Can you work these out from the drawing? Everything is in mm from the part's minimum corner. Coordinates: 2 decimals unless noted, no trailing zeros. Loops run counter-clockwise (first coordinate to the right, second up) from the corner with the lowest first, then second, coordinate; pieces in that order, holes last.
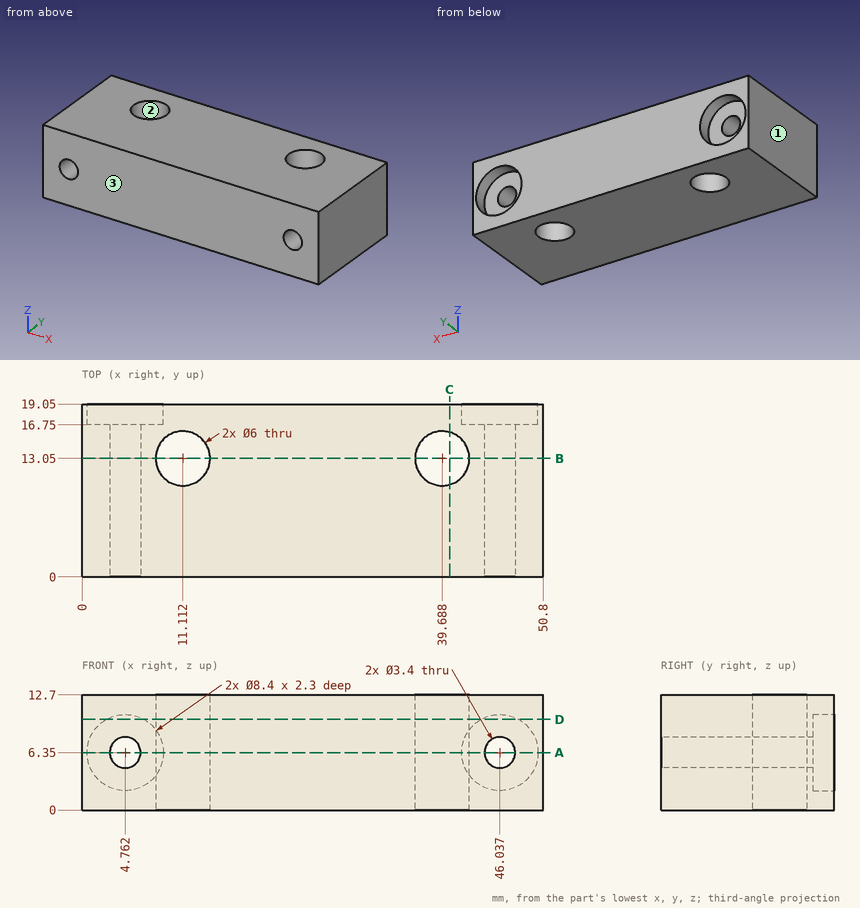
Item 1: I need wall thicknesses on line 1 along X through (y, z) = (2.75, 7.25) (1 decimal); line 2 along X through (y, z) = (14, 5.5) (1 decimal); line 3 along X through (y, z) = (18.25, 2.5) (1 decimal). Which ranges of each line are inside material? Lowest first, please.
Results are:
line 1: x = 0 to 3.3, 6.2 to 44.6, 47.5 to 50.8
line 2: x = 0 to 3.3, 6.2 to 8.3, 14 to 36.8, 42.5 to 44.6, 47.5 to 50.8
line 3: x = 0 to 3.1, 6.4 to 44.4, 47.7 to 50.8
Item 2: Suppose I cut it at A-A, the plane z = 6.35. Please give me the cut outline in (x, y).
Results are:
outline: (0, 0) - (3.06, 0) - (3.06, 16.75) - (0.56, 16.75) - (0.56, 19.05) - (0, 19.05) - close; (6.46, 0) - (44.34, 0) - (44.34, 16.75) - (41.84, 16.75) - (41.84, 19.05) - (8.96, 19.05) - (8.96, 16.75) - (6.46, 16.75) - close; (47.74, 0) - (50.8, 0) - (50.8, 19.05) - (50.24, 19.05) - (50.24, 16.75) - (47.74, 16.75) - close; hole circle Ø6 at (11.11, 13.05); hole circle Ø6 at (39.69, 13.05)
Item 3: Suppose I cut it at D-D, the plane z = 10. Count the separate pieces of the cut face and the enclosed holes in it, plus the area to 3 significant figures.
Results are:
separate pieces: 1
enclosed holes: 2
area: 892 mm2
Item 4: Suppose I cut it at C-C, the plane x = 40.5. Please give me the cut outline in (y, z).
Results are:
outline: (0, 0) - (10.16, 0) - (10.16, 12.7) - (0, 12.7) - close; (15.94, 0) - (19.05, 0) - (19.05, 12.7) - (15.94, 12.7) - close
Item 5: We'd pull the mould along Y, two halves only. Please class the marked faces 1, 2 and 3: +Y half, -Y half, draft (parallel to the pull), parting line (faces both ways), or undercut.
Results are:
face 1: draft
face 2: undercut
face 3: -Y half
Item 6: I'm going to push flat-ended pins straight in: P1, Ø9.5, axis at x = 39.69, y = 13.05, coming from the +Z side; P2, Ø4, axis at x = 45.5, z = 7, coming from the +Y side. Where does each tip first touch, or does it pass through?
Results are:
P1: stops at z = 12.7
P2: stops at y = 16.75
Item 7: Suppose I cut it at B-B, the plane y = 13.05. Please give me the cut outline in (x, z).
Results are:
outline: (0, 0) - (8.11, 0) - (8.11, 12.7) - (0, 12.7) - close; (14.11, 0) - (36.69, 0) - (36.69, 12.7) - (14.11, 12.7) - close; (42.69, 0) - (50.8, 0) - (50.8, 12.7) - (42.69, 12.7) - close; hole circle Ø3.4 at (4.76, 6.35); hole circle Ø3.4 at (46.04, 6.35)
